Job drawing, mm, ordinate dimensions from the low corner. One solid piece. Coordinates: 2 decimals unless noted, no trailing zeros. Order: outer loops, then holes, each group sorted by start corner. A loop starts at its lowest first (then second) coordinate and runs counter-clockwise, first axis right, second up. Notation, with made-up numbers: M 82,-15 L 99,-15 A29 ccw 99,13 Z; hole C 69.5,9.25 d4. An arc over 180 degrees is marked long. Write item = value, one per line.
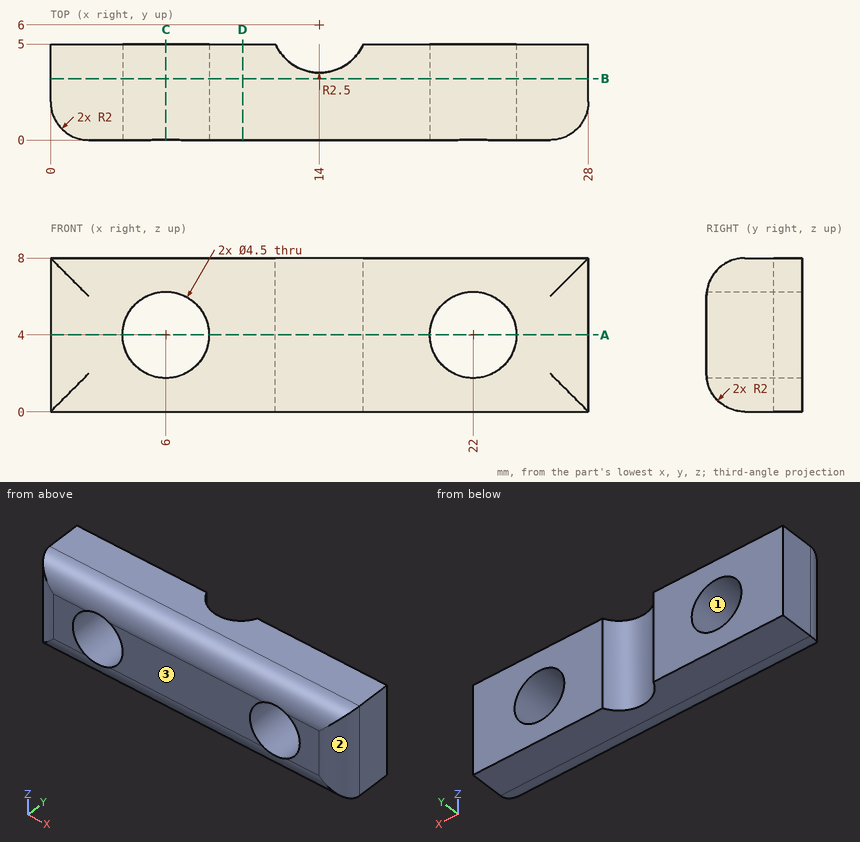
(1) Pull direction X, two halves, no side cores. Call the marked faces 1, 2 and 3: +X half, -X half, draft (parallel to the pull), parting line (faces both ways), or undercut.
Evaluation:
face_1 = undercut
face_2 = +X half
face_3 = draft
(2) Slice it at C-C, the plane x = 6. Write the cut outline in (y, z).
Evaluation:
outline = M 0.02,1.75 A2 ccw 2,0 L 5,0 L 5,1.75 Z; M 0.02,6.25 L 5,6.25 L 5,8 L 2,8 A2 ccw Z
(3) Slice it at D-D, the plane x = 10. Write the cut outline in (y, z), then the cut area to 3 significant figures.
Evaluation:
outline = M 0,2 A2 ccw 2,0 L 5,0 L 5,8 L 2,8 A2 ccw 0,6 Z
area = 38.3 mm²
(4) Wall check: line 1 (X direction, y = 2.3, z = 4); line 2 (X direction, y = 0.45, z = 5.25); line 3 (Z direction, x = 7, y = 3.4). Give the ranges that are in metal, low to high. Write a range as from..to.
Evaluation:
line_1 = 0..3.75, 8.25..19.75, 24.25..28
line_2 = 0.74..4.13, 7.87..20.13, 23.87..27.26
line_3 = 0..1.98, 6.02..8
(5) Slice it at B-B, the plane y = 3.2. Write the cut outline in (x, z), then the cut area to 3 significant figures.
Evaluation:
outline = M 0,0 L 28,0 L 28,8 L 0,8 Z; hole C 6,4 d4.5; hole C 22,4 d4.5
area = 192 mm²
(6) Slice it at A-A, the plane z = 4. Write the cut outline in (x, y), then the cut area to 3 significant figures.
Evaluation:
outline = M 0,2 A2 ccw 2,0 L 3.75,0 L 3.75,5 L 0,5 Z; M 8.25,0 L 19.75,0 L 19.75,5 L 16.29,5 A2.5 cw 11.71,5 L 8.25,5 Z; M 24.25,0 L 26,0 A2 ccw 28,2 L 28,5 L 24.25,5 Z
area = 88.3 mm²
